```python
from build123d import *

# Parameters (mm, degrees)
SKETCH1_R            = 44.45
BODY_EXTRUSION_DEPTH = 21.189302622
SKETCH6_R            = 3.81
DE_DEPTH             = 100
SKETCH7_R            = 7
INLET_TAP_DEPTH      = 8
BASE_START           = 5
SKETCH26_R           = 44.45
SKETCH26_R_2         = 22.09
BASE_RISER_DEPTH     = 5
SKETCH13_R           = 3
BOLT_HOLES_DEPTH     = 100
BOLT_PATTERN_COUNT   = 8


with BuildPart() as part:
    # Sketch1 → body extrusion (new body)
    with BuildSketch(Plane(origin=(0, 0, 0), x_dir=(1, 0, 0), z_dir=(0, 1, 0))):
        with Locations(Location((0, 0, 0), (0, 0, 270))):
            Circle(SKETCH1_R)
    extrude(amount=BODY_EXTRUSION_DEPTH)

    # Sketch2 → main chamber (revolve, cut)
    with BuildSketch(Plane.XY, mode=Mode.PRIVATE) as main_chamber_sk:
        Polygon((0, 0), (0, 9.189302622), (3.81, 9.189302622), (22.09, 4.5875), (22.09, 0), align=None)
    revolve(main_chamber_sk.sketch.rotate(Axis((0, 0, 0), (0, 1, 0)), 90), axis=Axis((0, 0, 0), (0, 1, 0)), mode=Mode.SUBTRACT)

    # Sketch6 → De (cut)
    with BuildSketch(Plane(origin=(0, 21.189302622, 0), x_dir=(1, 0, 0), z_dir=(0, 1, 0))):
        with Locations(Location((0, 0, 0), (0, 0, 270))):
            Circle(SKETCH6_R)
    extrude(amount=-DE_DEPTH, mode=Mode.SUBTRACT)

    # Sketch7 → inlet tap (cut)
    with BuildSketch(Plane(origin=(0, 21.189302622, 0), x_dir=(1, 0, 0), z_dir=(0, 1, 0))):
        with Locations(Location((0, 0, 0), (0, 0, 270))):
            Circle(SKETCH7_R)
    extrude(amount=-INLET_TAP_DEPTH, mode=Mode.SUBTRACT)

    # Sketch11 → conical outlet (revolve, cut)
    with BuildSketch(Plane(origin=(-5.360707244, 0, -20.006431798), x_dir=(0.9659258262890693, 0, -0.2588190451025173), z_dir=(0.2588190451025173, 0, 0.9659258262890693)), mode=Mode.PRIVATE) as conical_outlet_sk:
        Polygon((5.54981252, 4.401182844), (105.169282329, 13.116757119), (105.169282329, 3.79375), (5.54981252, 3.79375), align=None)
    revolve(conical_outlet_sk.sketch.rotate(Axis((0, 3.79375, -21.442828975), (0.9659258262890692, 0, -0.2588190451025173)), 255.191029346), axis=Axis((0, 3.79375, -21.442828975), (0.9659258262890692, 0, -0.2588190451025173)), mode=Mode.SUBTRACT)

    # Sketch16 → outer profile (revolve, cut)
    with BuildSketch(Plane.XY, mode=Mode.PRIVATE) as outer_profile_sk:
        Polygon((12, 21.189302622), (12, 12.956212983), (25.4, 9.582900339), (44.45, 9.582900339), (44.45, 21.189302622), align=None)
    revolve(outer_profile_sk.sketch.rotate(Axis((0, 0, 0), (0, 1, 0)), 90), axis=Axis((0, 0, 0), (0, 1, 0)), mode=Mode.SUBTRACT)

    # Sketch26 → base riser (add)
    with BuildSketch(Plane.XZ.offset(BASE_START)):
        with Locations(Location((0, 0, 0), (0, 0, 270))):
            Circle(SKETCH26_R)
        with Locations(Location((0, 0, 0), (0, 0, 270))):
            Circle(SKETCH26_R_2, mode=Mode.SUBTRACT)
    extrude(amount=-BASE_RISER_DEPTH)

    # Sketch13 → bolt holes (cut)
    with BuildSketch(Plane(origin=(0, 21.189302622, 0), x_dir=(1, 0, 0), z_dir=(0, 1, 0))):
        with Locations(Location((7.007261141, 34.214820127, 0), (0, 0, 90))):
            Circle(SKETCH13_R)
    bolt_holes = extrude(amount=-BOLT_HOLES_DEPTH, mode=Mode.SUBTRACT)

    # bolt pattern: bolt holes ×8 about axis
    bolt_pattern_axis = Axis((0, 0, 0), (0, 1, 0))
    for i in range(1, BOLT_PATTERN_COUNT):
        add(bolt_holes.rotate(bolt_pattern_axis, i * 360 / BOLT_PATTERN_COUNT), mode=Mode.SUBTRACT)


solid = part.part
```
Geometry: final body of the model. Coordinates: model frame, mm. A direction names the side the tool comes from. Coordinates: 2 decimals unless noted, no trailing zeros. Order: outer loops, then holes, each group sorted by start corner. A loop starts at its lowest first (then second) coordinate and runs counter-clockwise, first axis right, second up. Notation, with made-up numbers: (-22.75, 56) -> (17.25, 56) arc R21 cw to (17.25, 88) -> close; hole circle Ø10 at (5, -10.5). An arc over 180 degrees is marked (long way). Write item = value, one per line.
(1) Access query for faces 1 (the cylindrical face through (28.756, 2.394, -16.264)), 2 (the cylindrical face through (-3.604, 17.015, -11.446)). Directions: +Z, -Z, +X, -X, +Y, -Y. A direction counts if a zero-diameter tool reaches every point of the face in a straight line with its end or side. Return the directions, or none.
Solved:
face_1 = +Y, -Y
face_2 = +Y
(2) Cut plane A-A on z = 0. Return loops of the section in (x, y), plus the area to 3 significant figures.
Solved:
outline = (-44.45, -5) -> (-22.09, -5) -> (-22.09, 4.59) -> (-3.81, 9.19) -> (-3.81, 13.19) -> (-7, 13.19) -> (-7, 21.19) -> (-12, 21.19) -> (-12, 12.96) -> (-25.4, 9.58) -> (-44.45, 9.58) -> close; (3.81, 9.19) -> (22.09, 4.59) -> (22.09, -5) -> (44.45, -5) -> (44.45, 9.58) -> (25.4, 9.58) -> (12, 12.96) -> (12, 21.19) -> (7, 21.19) -> (7, 13.19) -> (3.81, 13.19) -> close
area = 935 mm²
(3) Pin query (flat end, axial travel): pin 1 Ø1 at (y, z) = (14.5, 1.5) entering from +X; pin 2 Ø2 at (x, z) = (-17, -12) entering from +Y; pin 3 Ø8 at (x, z) = (7.01, -34.21) entering from -Y; pin 4 Ø1 at (y, z) = (17.5, -10) entering from -X. Return the tip coordinate at first contact, or that it passes through.
Solved:
pin_1 = 11.96
pin_2 = 10.99
pin_3 = -5
pin_4 = -7.33
(4) Cut plane C-C on z = -38.5. Return loops of the section in (x, y).
Solved:
outline = (-22.22, -5) -> (22.22, -5) -> (22.22, 9.58) -> (-22.22, 9.58) -> close
(5) Pull-direction query (X, two-part tool) for faces 3 (the cylindrical face through (37.076, 2.394, 6.106)), 4 (the flat face through (19, 9.583, 19)), 5 (the conical face through (-3.856, 12.745, -12.245)), 6 (the flat face through (-3, 13.189, 3)); classes: pulls with the +X half, pulls with the -X half, needs draft (parallel to the pull), parting line crosses it, or undercut.
Solved:
face_3 = undercut
face_4 = needs draft
face_5 = parting line crosses it
face_6 = undercut
(6) Line query: line 1 (X direction, y = 16.25, z = 0); line 2 (X direction, y = 3.65, z = 0); line 3 (Y direction, x = -16, z = 34). Output: solid intervals per line, ascending.
Solved:
line_1 = -12 to -7, 7 to 12
line_2 = -44.45 to -22.09, 22.09 to 44.45
line_3 = -5 to 9.58
(7) Cut plane B-B on z = 28.5. Return loops of the section in (x, y).
Solved:
outline = (-34.11, -5) -> (16.31, -5) -> (16.31, 9.58) -> (-34.11, 9.58) -> close; (22.17, -5) -> (34.11, -5) -> (34.11, 9.58) -> (22.17, 9.58) -> close
